The model under review builds one solid part; all positions refer to its coordinate system, in mm. Round coordinates to 2 decimals unless told otherwise and drop trailing zeros. Write each loop counter-clockwise with the first axis right and the second up, starting at its lowest first coordinate (ties: lowest second). Pieces come first, ordered by that corner, then holes. Notation, with made-up numbers: M 88,22 L 108,22 A17 cw 108,35 Z; hole C -38,-39 d6. An arc over 180 degrees is marked long. One line per item, written item: value. Start each with the question number.
1) Take a section at A-A, the plane x = -20.5. Write out the cut boundary in (y, z).
2) Wall thickness on probe 1 along X at (y, z) = (0.95, 20.5); probe 2 along X at (y, z) = (0.65, -21.5): over which ranges is each line inside the solid? List them lowest first.
3) Take a section at B-B, the plane z = 20.5. Write out the cut boundary in (x, y).
4) For P1, Ø2.5, axis at x = -20.5, z = 20.5, coming from the -Y side, flat-tipped, find the tip position at first contact; note if it passes through.
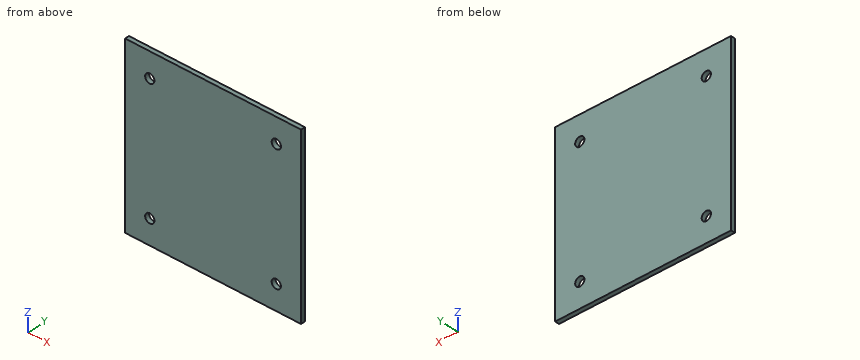
from build123d import *

# Parameters (mm, degrees)
SKETCH1_W           = 57
SKETCH1_H           = 57
SKETCH1_R           = 1.5
SKETCH1_W_2         = 25
SKETCH1_H_2         = 25
BOSS_EXTRUDE1_DEPTH = 1.397


with BuildPart() as part:
    # Sketch1 → Boss-Extrude1 (new body)
    # profile 1 of 2: a face of its own
    with BuildSketch(Plane(origin=(0, 0, 0), x_dir=(1, 0, 0), z_dir=(0, 1, 0))):
        Rectangle(SKETCH1_W, SKETCH1_H)
        with Locations(Location((-20.5, -20.5, 0), (0, 0, 270))):
            Circle(SKETCH1_R, mode=Mode.SUBTRACT)
        with Locations(Location((-20.5, 20.5, 0), (0, 0, 270))):
            Circle(SKETCH1_R, mode=Mode.SUBTRACT)
        with Locations(Location((20.5, -20.5, 0), (0, 0, 270))):
            Circle(SKETCH1_R, mode=Mode.SUBTRACT)
        with Locations(Location((20.5, 20.5, 0), (0, 0, 270))):
            Circle(SKETCH1_R, mode=Mode.SUBTRACT)
        Rectangle(SKETCH1_W_2, SKETCH1_H_2, mode=Mode.SUBTRACT)
    # profile 2 of 2: a face of its own
    with BuildSketch(Plane(origin=(0, 0, 0), x_dir=(1, 0, 0), z_dir=(0, 1, 0))):
        Rectangle(SKETCH1_W_2, SKETCH1_H_2)
    extrude(amount=BOSS_EXTRUDE1_DEPTH)


solid = part.part
Checked values:
1. outline: M 0,-28.5 L 1.4,-28.5 L 1.4,-22 L 0,-22 Z; M 0,-19 L 1.4,-19 L 1.4,19 L 0,19 Z; M 0,22 L 1.4,22 L 1.4,28.5 L 0,28.5 Z
2. probe 1: x = -28.5 to -22, -19 to 19, 22 to 28.5
2. probe 2: x = -28.5 to -21.62, -19.38 to 19.38, 21.62 to 28.5
3. outline: M -28.5,0 L -22,0 L -22,1.4 L -28.5,1.4 Z; M -19,0 L 19,0 L 19,1.4 L -19,1.4 Z; M 22,0 L 28.5,0 L 28.5,1.4 L 22,1.4 Z
4. P1: passes through
